```python
from build123d import *

# Parameters (mm, degrees)
SKETCH1_R           = 3
SKETCH1_R_2         = 1.6
BOSS_EXTRUDE1_DEPTH = 2.2
SKETCH1_3_R         = 1.6
BOSS_EXTRUDE2_DEPTH = 1
SKETCH5_R           = 1.5
BOSS_EXTRUDE3_DEPTH = 1
SKETCH6_R           = 2
BOSS_EXTRUDE4_DEPTH = 1
SKETCH8_R           = 1.5
BOSS_EXTRUDE5_DEPTH = 3


with BuildPart() as part:
    # Sketch1 → Boss-Extrude1 (new body)
    with BuildSketch(Plane(origin=(0, 0, 0), x_dir=(1, 0, 0), z_dir=(0, 1, 0))):
        with Locations((-0.522013312, 0.511138034)):
            Circle(SKETCH1_R)
        with Locations((-0.522013312, 0.511138034)):
            Circle(SKETCH1_R_2, mode=Mode.SUBTRACT)
    extrude(amount=BOSS_EXTRUDE1_DEPTH)

    # Sketch1<3> → Boss-Extrude2 (add)
    with BuildSketch(Plane(origin=(0, 0, 0), x_dir=(1, 0, 0), z_dir=(0, 1, 0))):
        with Locations((-0.522013312, 0.511138034)):
            Circle(SKETCH1_3_R)
    extrude(amount=BOSS_EXTRUDE2_DEPTH)

    # Sketch5 → Boss-Extrude3 (add)
    with BuildSketch(Plane.XZ):
        with Locations((-0.522013312, -0.511138034)):
            Circle(SKETCH5_R)
    extrude(amount=BOSS_EXTRUDE3_DEPTH)

    # Sketch6 → Boss-Extrude4 (add)
    with BuildSketch(Plane.XZ.offset(1)):
        with Locations((-0.522013312, -0.511138034)):
            Circle(SKETCH6_R)
    extrude(amount=BOSS_EXTRUDE4_DEPTH)

    # Sketch8 → Boss-Extrude5 (add)
    with BuildSketch(Plane(origin=(0, -2, 0), x_dir=(-1, 0, 0), z_dir=(0, -1, 0))):
        with Locations((0.522013312, 0.511138034)):
            Circle(SKETCH8_R)
    extrude(amount=BOSS_EXTRUDE5_DEPTH)


solid = part.part
```
Work out the finished part from the listing and answer in its coordinate system (mm). A direction names the side the tool comes from. Round coordinates to 2 decimals unless told otherwise and drop trailing zeros. Write each loop counter-clockwise with the first axis right and the second up, starting at its lowest first coordinate (ties: lowest second). Pieces come first, ordered by that corner, then holes. Notation, with made-up numbers: (-5.75, -10.75) -> (46.25, -10.75) arc R28 ccw to (46.25, 8.25) -> close; hole circle Ø4 at (-24, 18.5). An arc over 180 degrees is marked (long way). Write each question's results on one line, items separated by ' | '.
Q1. Section D-D, the plane x = -1.45 is taken. Write down the section's boundary in (y, z), then the cut area to 3 significant figures.
Data:
outline: (-5, -1.69) -> (-2, -1.69) -> (-2, -2.28) -> (-1, -2.28) -> (-1, -1.69) -> (0, -1.69) -> (0, -3.36) -> (2.2, -3.36) -> (2.2, -1.81) -> (1, -1.81) -> (1, 0.79) -> (2.2, 0.79) -> (2.2, 2.34) -> (0, 2.34) -> (0, 0.67) -> (-1, 0.67) -> (-1, 1.26) -> (-2, 1.26) -> (-2, 0.67) -> (-5, 0.67) -> close | area: 22.4 mm^2
Q2. Determine the mould class of faces 4 (the cylindrical face through (-0.197, -3.479, 0.953)), 5 (the cylindrical face through (1, 2, -1)), 6 (the flat face through (-1, -5, -1)), 7 (the flat face through (-1, 1, -1)) for opening direction X: released by +X, released by -X, zero draft, split by the parting line, or undercut.
Data:
face 4: split by the parting line | face 5: undercut | face 6: zero draft | face 7: undercut
Q3. Flat-ended cylindrical pins translate along their axes: P1, Ø1, axis at x = -1.5, y = 1, coming from the -Z side; P2, Ø1.5, axis at y = 1, z = 0.5, coming from the -X side; P3, Ø2.5, axis at x = -1, z = -1, coming from the +Y side. Find the tip coordinate at first contact, or state that the pin passes through.
Data:
P1: z = -3.47 | P2: x = -3.51 | P3: y = 2.2
Q4. Which of the six approach directions +Z, -Z, +X, -X, +Y, -Y give full straight-line access (tool end or side, diameter ignored) to faces 1 (the flat face through (1, 0, 1)), 2 (the cylindrical face through (-1.17, 1.08, 2.42)), 3 (the cylindrical face through (1.325, -1.493, -1.277))?
Data:
face 1: none | face 2: +Y, -Y | face 3: -Y
Q5. Section A-A, the plane z = -2.25 is taken. Write down the section's boundary in (x, y), then the cut area to 3 significant figures.
Data:
outline: (-2.97, 0) -> (1.92, 0) -> (1.92, 2.2) -> (-2.97, 2.2) -> close; (-1.51, -2) -> (0.47, -2) -> (0.47, -1) -> (-1.51, -1) -> close | area: 12.7 mm^2
Q6. Section C-C, the plane z = -1.6 is taken. Write down the section's boundary in (x, y), then the cut area to 3 significant figures.
Data:
outline: (-3.32, 0) -> (-1.55, 0) -> (-1.55, -1) -> (-2.2, -1) -> (-2.2, -2) -> (-1.55, -2) -> (-1.55, -5) -> (0.51, -5) -> (0.51, -2) -> (1.16, -2) -> (1.16, -1) -> (0.51, -1) -> (0.51, 0) -> (2.27, 0) -> (2.27, 2.2) -> (0.65, 2.2) -> (0.65, 1) -> (-1.69, 1) -> (-1.69, 2.2) -> (-3.32, 2.2) -> close | area: 21.1 mm^2
Q7. Section B-B, the plane x = 1.3 is taken. Write down the section's boundary in (y, z), then the cut area to 3 significant figures.
Data:
outline: (-2, -1.34) -> (-1, -1.34) -> (-1, 0.31) -> (-2, 0.31) -> close; (0, -2.89) -> (2.2, -2.89) -> (2.2, 1.87) -> (0, 1.87) -> close | area: 12.1 mm^2
Q8. Straight lines are drawn through the part: line 1 along Y through (x, z) = (0.45, -1.7); line 2 along Y through (x, z) = (1.25, 1.75); line 3 along Y through (x, z) = (0.3, 1). For each, find the intervals that lie inside material, in ascending order. Write a range as [from, to].
Data:
line 1: [-2, -1], [0, 1] | line 2: [0, 2.2] | line 3: [-2, -1], [0, 2.2]
